Answer from the drawing. Dimensions are ordinates in mm from the lowest x, y and z of the part. Round coordinates to 2 decimals unless told otherwise and drop trailing zeros. Order: outer loops, then holes, each group sorted by start corner. A loop starts at its lowest first (then second) coordinate and runs counter-clockwise, first axis right, second up. Notation, with made-up numbers: (54, 31) -> (90, 31) arc R18 cw to (90, 59) -> close; hole circle Ø2 at (-34, -1.75). An arc over 180 degrees is marked (long way). Use a Markdown table: item, result. Add a question column.
Item 1: Find the intervals of material crossed by L1, parallel to Z at x = 105, y = 6.5; L2, parallel to Y at x = 7.5, z = 5; L3, parallel to X at y = 11.25, z = 5, in increasing order. Write a range as [from, to].
Item 2: Flat-ended cylindrical pins translate along their axes: P1, Ø6, axis at y = 106.5, z = 1, coming from the +X side; P2, Ø5.5, axis at x = 105, z = 5.5, coming from the -Y side; P3, Ø3, axis at x = 105, z = 5, coming from the +Y side; P4, Ø1.6, axis at y = 105, z = 5, coming from the -X side. Find the tip coordinate at first contact, or state that the pin passes through.
Item 3: A cutting plane is placed at C-C, the plane x = 9. Determine the outline of the cut face in (y, z), plus the area to 3 significant figures.
Item 4: A cutting plane is placed at A-A, the plane y = 40. Determine the outline of the cut face in (x, z).
Item 5: A cutting plane is placed at B-B, the plane z = 5. Determine the outline of the cut face in (x, y).
Item 6: A cutting plane is placed at D-D, the plane x = 105. Determine the outline of the cut face in (y, z), plus the area to 3 significant figures.
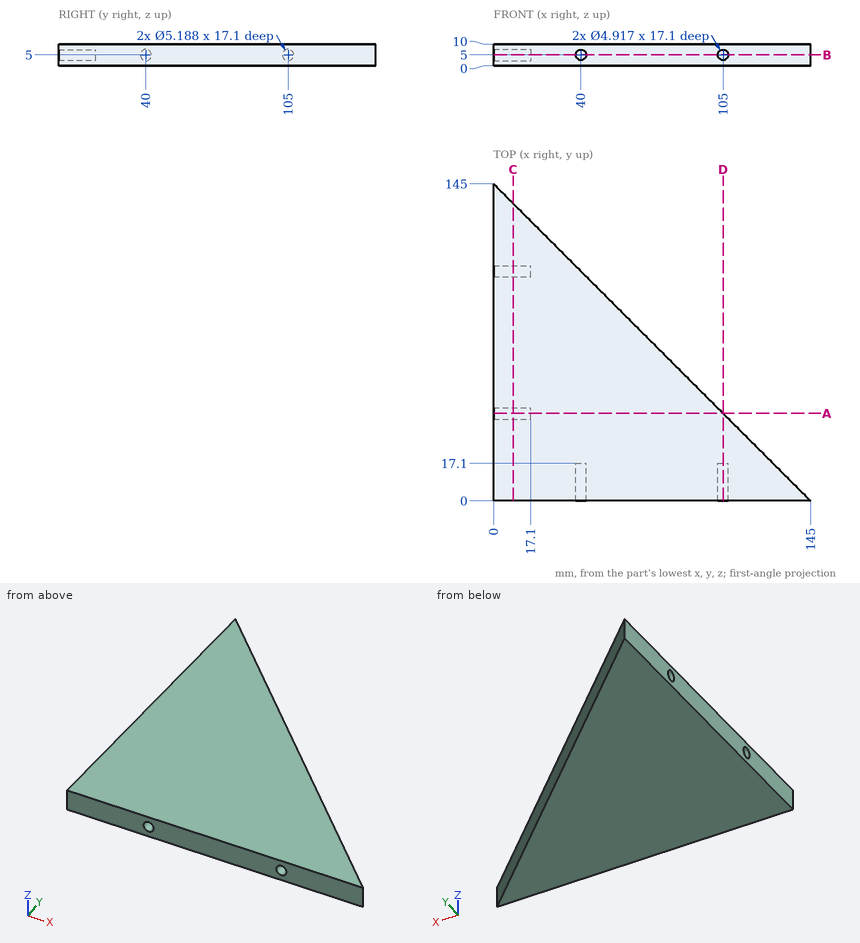
Reported:
| question | item | result |
|---|---|---|
| 1 | L1 | [0, 2.54], [7.46, 10] |
| 1 | L2 | [0, 37.41], [42.59, 102.41], [107.59, 137.5] |
| 1 | L3 | [0, 37.54], [42.46, 102.54], [107.46, 133.75] |
| 2 | P1 | x = 41.5 |
| 2 | P2 | y = 0 |
| 2 | P3 | y = 41.5 |
| 2 | P4 | x = 17.1 |
| 3 | outline | (0, 0) -> (136, 0) -> (136, 10) -> (0, 10) -> close; hole circle Ø5.19 at (40, 5); hole circle Ø5.19 at (105, 5) |
| 3 | area | 1,320 mm² |
| 4 | outline | (0, 0) -> (105, 0) -> (105, 10) -> (0, 10) -> (0, 7.59) -> (17.1, 7.59) -> (17.1, 2.41) -> (0, 2.41) -> close |
| 5 | outline | (0, 0) -> (37.54, 0) -> (37.54, 17.1) -> (42.46, 17.1) -> (42.46, 0) -> (102.54, 0) -> (102.54, 17.1) -> (107.46, 17.1) -> (107.46, 0) -> (145, 0) -> (0, 145) -> (0, 107.59) -> (17.1, 107.59) -> (17.1, 102.41) -> (0, 102.41) -> (0, 42.59) -> (17.1, 42.59) -> (17.1, 37.41) -> (0, 37.41) -> close |
| 6 | outline | (0, 0) -> (40, 0) -> (40, 10) -> (0, 10) -> (0, 7.46) -> (17.1, 7.46) -> (17.1, 2.54) -> (0, 2.54) -> close |
| 6 | area | 316 mm² |
